The drawing under review shows one solid part. Ordinate dimensions are in mm from its lowest x, y, z. A direction names the side the tool comes from. Coordinates: 2 decimals unless noted, no trailing zeros. Loops run counter-clockwise (first coordinate to the right, second up) from the corner with the lowest first, then second, coordinate; pieces in that order, holes last. Notation, with made-up numbers: (65.5, -18.5) - (73.5, -18.5) arc R26 ccw to (73.5, 16.5) - close; hole circle Ø6 at (-39.5, 34.25). An arc over 180 degrees is marked (long way). Answer as a JSON object with one key per item and string values. Group by question number.
Item 1: To check wall thickness, follow line 1 (Y direction, x = 19, z = 7.5); line 2 (Z direction, x = 20.25, y = 51.5); line 3 (Z direction, x = 4.25, y = 61). State the ranges of each line that lie inside material, in increasing order.
Item 2: We need section B-B (z = 47.5). Give the boundary of the cut face in (x, y).
Item 3: We need section D-D (y = 41). Give the boundary of the cut face in (x, z).
Item 4: We need section C-C (x = 12.7). Give the boundary of the cut face in (y, z).
Item 5: Clearance check with flat-ended pins moving along their axes: pin 1 (1 mm diameter, centred on x = 2.5, y = 40, fed in from +Z); pin 2 (12 mm diameter, centred on x = 19, y = 103.5, fed in from +Z); pin 3 (6 mm diameter, centred on x = 20.5, y = 34.5, fed in from +Z). State where each tip first meets the part, or that it passes through.
Item 6: We need section A-A (y = 20). Give the boundary of the cut face in (x, z), then the cut area to 3 significant figures.
Item 7: Tool access review of the marked faces 1 and 2: name each direction out of +Z, -Z, +X, -X, +Y, -Y from which nothing blocks a thin tool from reaching the whole face with its end or side.
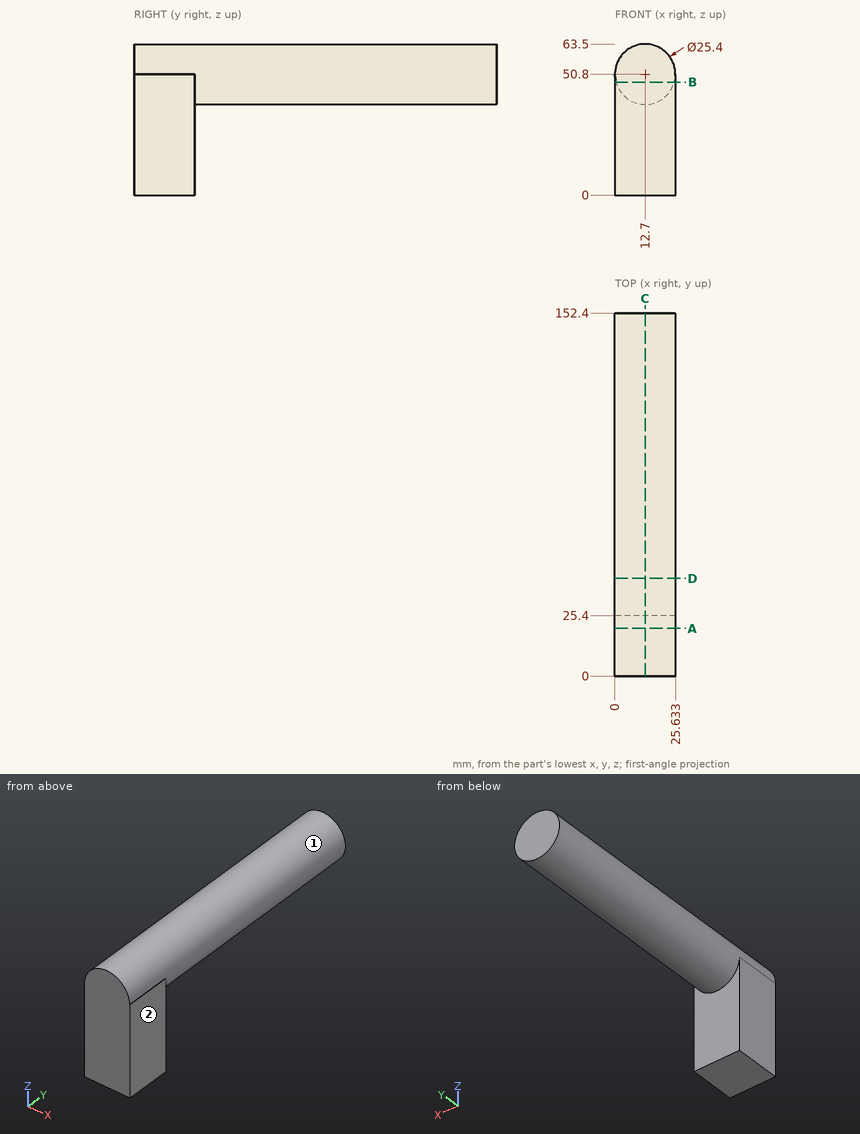
Check sheet entries:
{
 "1": {"line 1": "y = 0 to 25.4", "line 2": "z = 40.59 to 61.01", "line 3": "z = 41.32 to 60.28"},
 "2": {"outline": "(0, 0) - (25.63, 0) - (25.63, 25.4) - (24.96, 25.4) - (24.96, 152.4) - (0.44, 152.4) - (0.44, 25.4) - (0, 25.4) - close"},
 "3": {"outline": "circle Ø25.4 at (12.7, 50.8)"},
 "4": {"outline": "(0, 0) - (25.4, 0) - (25.4, 38.1) - (152.4, 38.1) - (152.4, 63.5) - (0, 63.5) - close"},
 "5": {"pin 1": "stops at z = 59", "pin 2": "stops at z = 63.5", "pin 3": "stops at z = 62.56"},
 "6": {"outline": "(0, 0) - (25.63, 0) - (25.63, 50.8) - (25.4, 50.8) arc R12.7 ccw to (0, 50.8) - close", "area": "1,560 mm2"},
 "7": {"face 1": "+Y", "face 2": "+Z, -Z, +X, +Y, -Y"}
}
